Autodesk Inventor part; units mm, degrees
ref_plane "Work Plane1" through (0, 62.4, 0) normal (0, 1, 0) x (1, 0, 0)
ref_plane "YZ Plane" through (0, 0, 0) normal (1, 0, 0) x (0, 1, 0)
ref_plane "XZ Plane" through (0, 0, 0) normal (0, 1, 0) x (-1, 0, 0)
sketch "Sketch1" plane through (0, 0, 0) normal (0, 1, 0) x (-1, 0, 0)
  circle A0 centre (0, 0) radius 18
  dimension "d0" = 36
extrude "Extrusion1" add sketch "Sketch1" along normal blind 65
ref_plane "Work Plane1" through (0, 62.4, 0) normal (0, 1, 0) x (1, 0, 0)
sketch "Sketch2" plane through (0, 62.4, 0) normal (0, 1, 0) x (1, 0, 0)
  circle A0 centre (0, 0) radius 18
  circle A1 centre (0, 0) radius 19.4
  line L0 (-15.5, -1.35) -> (-20.5, -1.35)
  line L1 (-20.5, -1.35) -> (-20.5, 1.35)
  line L2 (-20.5, 1.35) -> (-15.5, 1.35)
  line L3 (-15.5, 1.35) -> (-15.5, -1.35)
  circle A2 centre (0, 0) radius 18
  line L4 (-15.5, -1.35) -> (-20.5, 1.35) construction
  line L5 (-20.5, -1.35) -> (-15.5, 1.35) construction
  point P0 (-18, 0)
  point P1 (-19.353, 1.35)
  point P2 (-17.9493, 1.35)
  point P3 (-17.9493, -1.35)
  point P4 (-19.353, -1.35)
  dimension "d4" = 38.8
  dimension "d5" = 5
  dimension "d6" = 2.7
extrude "Extrusion2" add sketch "Sketch2" against normal blind 50 contours A0 L2 A1 L0 picked at (18.5875, 2.9161)
sketch "Sketch3" plane through (0, 65, 0) normal (0, 1, 0) x (1, 0, 0)
  circle A0 centre (0, 0) radius 18
  circle A1 centre (0, 0) radius 6.5
  dimension "d9" = 13
extrude "Extrusion3" add sketch "Sketch3" along normal blind 4.5 contours A1
sketch "Sketch4" plane through (0, 0, 0) normal (0, -1, 0) x (1, 0, 0)
  circle A0 centre (0, 0) radius 18
  circle A1 centre (0, 0) radius 5.1
  dimension "d12" = 10.2
extrude "Extrusion4" add sketch "Sketch4" along normal blind 3.4 contours A1
sketch "Sketch5" plane through (0, 65, 0) normal (0, 1, 0) x (1, 0, 0)
  circle A0 centre (0, 0) radius 6.5
  circle A1 centre (0, 0) radius 18
  line L0 (0, 0) -> (0, -12.5)
  line L1 (0, 0) -> (0, 12.5)
  circle A2 centre (0, -12.5) radius 1.5
  circle A3 centre (0, 12.5) radius 1.5
  dimension "d15" = 12.5
  dimension "d16" = 12.5
  dimension "d17" = 3
  dimension "d18" = 3
extrude "Extrusion5" cut sketch "Sketch5" against normal blind 3 contours A2 | A3
sketch "Sketch6" plane through (0, 65, 0) normal (0, 1, 0) x (1, 0, 0)
  circle A0 centre (0, 0) radius 6.5
  line L0 (10.5, 10.5) -> (-10.5, 10.5)
  line L1 (-10.5, 10.5) -> (-10.5, -10.5)
  line L2 (-10.5, -10.5) -> (10.5, -10.5)
  line L3 (10.5, -10.5) -> (10.5, 10.5)
  circle A1 centre (0, 0) radius 5.1
  line L4 (10.5, 10.5) -> (-10.5, -10.5) construction
  line L5 (-10.5, 10.5) -> (10.5, -10.5) construction
  circle A2 centre (10.5, -10.5) radius 1
  circle A3 centre (-10.5, -10.5) radius 1
  circle A4 centre (-10.5, 10.5) radius 1
  circle A5 centre (10.5, 10.5) radius 1
  dimension "d21" = 21
  dimension "d22" = 21
  dimension "d23" = 2
  dimension "d24" = 2
  dimension "d25" = 2
  dimension "d26" = 2
extrude "Extrusion6" cut sketch "Sketch6" against normal blind 1 contours A4 L1 L0 | L0 L1 A4 | A5 L3 L0 | L0 L3 A5 | A3 L2 L1 | L1 L2 A3 | A2 L2 L3 | L3 L2 A2
sketch "Sketch7" plane through (0, 65, 0) normal (0, 1, 0) x (1, 0, 0)
  circle A0 centre (0, 0) radius 6.5
  circle A1 centre (0, 0) radius 1.5875
  dimension "d29" = 3.175
extrude "Extrusion7" add sketch "Sketch7" against normal blind 76.2 contours A1
sketch "Sketch8" plane through (0, -11.2, 0) normal (0, -1, 0) x (1, 0, 0)
  circle A0 centre (0, 0) radius 1.5875
extrude "Extrusion8" add sketch "Sketch8" against normal blind 100
sketch "Sketch9" plane through (0, 0, 0) normal (0, -1, 0) x (1, 0, 0)
  circle A0 centre (0, 0) radius 5.1
  circle A1 centre (0, 0) radius 18
  circle A2 centre (0, 0) radius 1.5875
  line L0 (0, 0) -> (19.2, 0)
  line L1 (16.8, -3.75) -> (19.2, -3.75)
  line L2 (19.2, -3.75) -> (19.2, 3.75)
  line L3 (19.2, 3.75) -> (16.8, 3.75)
  line L4 (16.8, 3.75) -> (16.8, -3.75)
  circle A3 centre (0, 0) radius 18
  line L5 (16.8, -3.75) -> (19.2, 3.75) construction
  line L6 (19.2, -3.75) -> (16.8, 3.75) construction
  point P0 (18, 0)
  dimension "d34" = 19.2
  dimension "d35" = 2.4
  dimension "d36" = 7.5
extrude "Extrusion9" add sketch "Sketch9" against normal blind 5 contours L4 L3 A1 L0 | L0 A1 L1 L4 | L0 L2 L1 A1 | A1 L3 L2 L0
chamfer "Chamfer1" distance 1 angle 45 2 edges at (19.2, 2.5, -3.75) (19.2, 2.5, 3.75)
sketch "Sketch10" plane through (0, 0, 0) normal (0, -1, 0) x (1, 0, 0)
  line L0 (19.2, 2.75) -> (18.2, 3.75)
  line L1 (19.2, 2.75) -> (19.2, -2.75)
  line L2 (18.2, -3.75) -> (19.2, -2.75)
  line L3 (18.2, -3.75) -> (17.605, -3.75)
  arc A0 (17.605, -3.75) -> (17.605, 3.75) centre (0, 0) ccw
  line L4 (17.605, 3.75) -> (18.2, 3.75)
extrude "Extrusion10" cut sketch "Sketch10" against normal blind 1
properties part number "motor_1"
Source: CAD feature listing. Evaluate the final solid. Frame: model axes, mm. A direction names the side the tool comes from. Give positions to 0.01 mm unless a question says otherwise; leave off trailing zeros. Write each loop counter-clockwise with the first axis right and the second up, starting at its lowest first coordinate (ties: lowest second). Pieces come first, ordered by that corner, then holes.
1. Pull-direction query (X, two-part tool) for faces 4 (the face through (-0.34, -7.25, 1.55)), 5 (the face through (0, 62, 12)), 6 (the face through (17.2, 62.4, -5.8)); classes: +X half, -X half, draft (parallel to the pull), parting line (faces both ways), or undercut.
2. Access query for faces 1 (the face through (0, 88.8, 0)), 2 (the face through (-4, 0, -4)), 3 (the face through (0, 62, -13)). Directions: +Z, -Z, +X, -X, +Y, -Y. A direction counts if a zero-diameter tool reaches every point of the face in a straight line with its end or side. Return the directions, or none.
3. Material intervals for line 1 along Z through (x, y) = (0, 62.95); line 2 along X through (y, z) = (64.75, -10.5); line 3 along Y through (x, z) = (3.5, 0.5), sorted ascending.
4. Section query B-B (z = -15). Return the cut outline in (x, y), then the cut area to 3 significant figures.
5. First-contact query: pin 1 (0.6 mm diameter, centred on x = -10.5, z = 11, fed in from +Y); pin 2 (8 mm diameter, centred on y = 34.5, z = -5.5, fed in from -X); pin 3 (4 mm diameter, centred on x = 9.5, y = 12, fed in from -Z). Flat tips, straight axial feed; report the tip coordinate or a pass-through.
6. Section query D-D (x = 2.5). Return the cut outline in (y, z), then the cut area to 3 significant figures.
7. Section query C-C (y = 75). Return the cut outline in (x, z) (1 decimal), then the cut area to 3 significant figures.
8. Section query A-A (x = 10.5). Return the cut outline in (y, z).
Output values:
1. face 4: parting line
1. face 5: undercut
1. face 6: draft
2. face 1: +Z, -Z, +X, -X, +Y
2. face 2: -Y
2. face 3: +Y
3. line 1: z = -18 to -14, -11 to 11, 14 to 18
3. line 2: x = -14.62 to -11.5, -9.5 to 9.5, 11.5 to 14.62
3. line 3: y = -3.4 to 69.5
4. outline: (-12.3, 12.4) - (-9.95, 12.4) - (-9.95, 0) - (9.95, 0) - (9.95, 12.4) - (12.3, 12.4) - (12.3, 62.4) - (9.95, 62.4) - (9.95, 65) - (-9.95, 65) - (-9.95, 62.4) - (-12.3, 62.4) - close
4. area: 1,530 mm2
5. pin 1: stops at y = 64
5. pin 2: stops at x = -19.34
5. pin 3: stops at z = -17.87
6. outline: (-3.4, -4.45) - (0, -4.45) - (0, -17.83) - (12.4, -17.83) - (12.4, -19.24) - (62.4, -19.24) - (62.4, -17.83) - (65, -17.83) - (65, -6) - (69.5, -6) - (69.5, 6) - (65, 6) - (65, 17.83) - (62.4, 17.83) - (62.4, 19.24) - (12.4, 19.24) - (12.4, 17.83) - (0, 17.83) - (0, 4.45) - (-3.4, 4.45) - close
6. area: 2,540 mm2
7. outline: circle Ø3.2 at (0, 0)
7. area: 7.92 mm2
8. outline: (0, -14.62) - (12.4, -14.62) - (12.4, -16.31) - (62.4, -16.31) - (62.4, -14.62) - (65, -14.62) - (65, -11.5) - (64, -11.5) - (64, -9.5) - (65, -9.5) - (65, 9.5) - (64, 9.5) - (64, 11.5) - (65, 11.5) - (65, 14.62) - (62.4, 14.62) - (62.4, 16.31) - (12.4, 16.31) - (12.4, 14.62) - (0, 14.62) - close
